from build123d import *

# Parameters (mm, degrees)
SKETCH_1_W                  = 35.1
SKETCH_1_H                  = 36.1
EXTRUDE_1_DEPTH             = 4.5
CHAMFER_1_SIZE              = 2
HOLE_WIZARD_M41_D           = 4.5
HOLE_WIZARD_M41_CSINK_D     = 4.55
HOLE_WIZARD_M41_CSINK_ANGLE = 90


with BuildPart() as part:
    # Эскиз1 → Бобышка-Вытянуть1 (new body)
    with BuildSketch(Plane.XY):
        Rectangle(SKETCH_1_W, SKETCH_1_H)
    extrude(amount=EXTRUDE_1_DEPTH)

    # Фаска1
    chamfer_1_edges = [part.edges().sort_by_distance(p)[0] for p in [
        (17.55, -18.05, 2.25),
        (-17.55, -18.05, 2.25),
        (-17.55, 18.05, 2.25),
        (17.55, 18.05, 2.25),
    ]]
    chamfer(chamfer_1_edges, length=CHAMFER_1_SIZE)

    # Отверстие с зазором M41 (through all)
    with Locations(Plane(origin=(-14.5, 15, 4.5), x_dir=(1, 0, 0), z_dir=(0, 0, 1))):
        with Locations((0, 0), (29, 0), (29, -30), (0, -30)):
            CounterSinkHole(HOLE_WIZARD_M41_D / 2, HOLE_WIZARD_M41_CSINK_D / 2, counter_sink_angle=HOLE_WIZARD_M41_CSINK_ANGLE)


solid = part.part
The listing builds one solid part. Answer for the finished solid, in the listing's coordinates (mm). Give positions to 0.01 mm unless a question says otherwise; leave off trailing zeros. Write each loop counter-clockwise with the first axis right and the second up, starting at its lowest first coordinate (ties: lowest second). Pieces come first, ordered by that corner, then holes.
Item 1: Section A-A, the plane y = -15 is taken. Write down the section's boundary in (x, z) (3 decimals).
Item 2: Section C-C, the plane z = 2.65 is taken. Write down the section's boundary in (x, y), plus the area to 3 significant figures.
Item 3: Determine the mould class of faces 1 (the flat face through (0, -18.05, 2)), 2 (the cylindrical face through (-15.538, 13.004, 2.206)), 3 (the flat face through (0, 18.05, 2)) for opening direction Y: released by +Y, released by -Y, zero draft, split by the parting line, or undercut.
Item 4: Find the intervals of material crossed by line 1 along X through (y, z) = (-15, 1.3); line 2 along Y through (x, z) = (14.5, 3.55); line 3 along X through (y, z) = (16, 2.4), in increasing order.
Item 5: Section B-B, the plane x = 14.5 is taken. Write down the section's boundary in (y, z) (3 decimals).
Completed:
1. outline: (-17.55, 0) - (-16.75, 0) - (-16.75, 4.475) - (-16.775, 4.5) - (-17.55, 4.5) - close; (-12.25, 0) - (12.25, 0) - (12.25, 4.475) - (12.225, 4.5) - (-12.225, 4.5) - (-12.25, 4.475) - close; (16.75, 0) - (17.55, 0) - (17.55, 4.5) - (16.775, 4.5) - (16.75, 4.475) - close
2. outline: (-17.55, -16.05) - (-15.55, -18.05) - (15.55, -18.05) - (17.55, -16.05) - (17.55, 16.05) - (15.55, 18.05) - (-15.55, 18.05) - (-17.55, 16.05) - close; hole circle Ø4.5 at (-14.5, -15); hole circle Ø4.5 at (-14.5, 15); hole circle Ø4.5 at (14.5, -15); hole circle Ø4.5 at (14.5, 15)
2. area: 1,200 mm2
3. face 1: released by -Y
3. face 2: undercut
3. face 3: released by +Y
4. line 1: x = -17.55 to -16.75, -12.25 to 12.25, 16.75 to 17.55
4. line 2: y = -18.05 to -17.25, -12.75 to 12.75, 17.25 to 18.05
4. line 3: x = -17.55 to -16.52, -12.48 to 12.48, 16.52 to 17.55
5. outline: (-18.05, 0) - (-17.25, 0) - (-17.25, 4.475) - (-17.275, 4.5) - (-18.05, 4.5) - close; (-12.75, 0) - (12.75, 0) - (12.75, 4.475) - (12.725, 4.5) - (-12.725, 4.5) - (-12.75, 4.475) - close; (17.25, 0) - (18.05, 0) - (18.05, 4.5) - (17.275, 4.5) - (17.25, 4.475) - close
